Design review of the part built by this model. Coordinates are the model's own, in mm. Face numbers are marked on the shaded views. A direction names the side the tool comes from. Give positions to 0.01 mm unless a question says otherwise; leave off trailing zeros. Order: outer loops, then holes, each group sorted by start corner. A loop starts at its lowest first (then second) coordinate and runs counter-clockwise, first axis right, second up. Notation, with made-up numbers: (29, 4.25) -> (47, 4.25) arc R25 cw to (47, 32.25) -> close; hole circle Ø4 at (62, 17.5). An arc over 180 degrees is marked (long way). One line per item, written item: value. Start each with the question number.
1) The part is to be moulded in two halves that separate along X. For the marked faces 1, 2, 3 and 4, say which applies: released by +X, released by -X, zero draft, split by the parting line, or undercut.
2) Consider section A-A (x = -0.25). State the section outline as (y, z) points.
3) Consider section C-C (z = 3.5). State the section outline as (x, y) points (3 decimals), plus the area to 3 significant figures.
4) Consider section D-D (z = 23.5). State the section outline as (x, y) points (3 decimals).
5) Wall thickness on line 1 along X through (y, z) = (9, 1.75); line 2 along Z through (x, y) = (8.25, 25); line 3 along Y through (x, z) = (0.5, 7.25): over which ranges is each line inside the solid? List them lowest first. Write a range as from..to.
6) Tool access review of the marked faces 5 and 6: name each direction out of +Z, -Z, +X, -X, +Y, -Y from which nothing blocks a thin tool from reaching the whole face with its end or side.
7) For pin 1 (10 mm diameter, centred on x = 1.5, y = 11, fed in from +Z); pin 2 (1.1 mm diameter, centred on x = 11, z = 27, fed in from -Y) (3 decimals); pin 3 (1.9 mm diameter, centred on x = -4.5, z = 28, fed in from +Y) (3 decimals), all flat-tipped, find the tip position at first contact; note any pin that passes through.
8) Consider section B-B (y = 2.95). State the section outline as (x, z) points, plus the area to 3 significant figures.
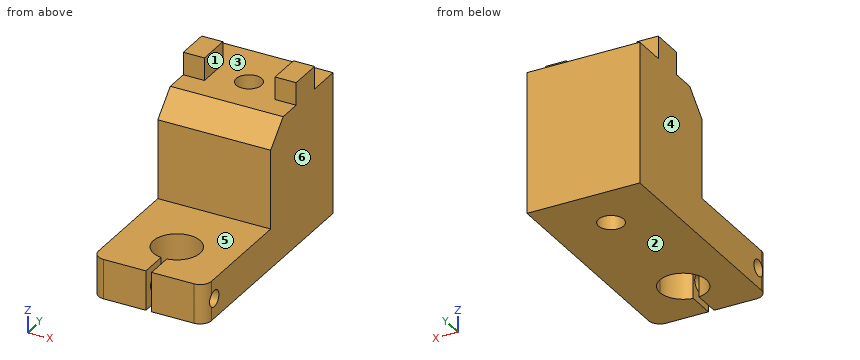
from build123d import *

# Parameters (mm, degrees)
F1_DEPTH    = 7
F2_R        = 1.45
F3_DEPTH    = 25
F4_T1_DEPTH = 17
F5_DEPTH    = 25
F0_W        = 3.75
F0_H        = 5.9
F6_DEPTH    = 29
F7_SIZE     = 4


# Not quite as in the source:
# - a fillet or chamfer that OpenCascade refuses, or shapes differently, is made with other operations: its cross-section is extruded or revolved along the edge and cut away or added
# - a feature names something its author has since deleted; it is built from what else it names


with BuildPart() as f1:
    # F0 (on Top) → F1 (new body)
    with BuildSketch(Plane.XY):
        Polygon((-6.5963959517, 29.175), (-6.5963959517, 21), (13.4036040483, 21), (13.4036040483, 29.175), (9.6536040483, 29.175), (9.6536040483, 35.075), (13.4036040483, 35.075), (13.4036040483, 41), (-6.5963959517, 41), (-6.5963959517, 35.075), (-2.8463959517, 35.075), (-2.8463959517, 29.175), align=None)
        with BuildLine():
            ThreePointArc((1.1536040483, 32.125), (3.4036040483, 34.375), (5.6536040483, 32.125))
            ThreePointArc((5.6536040483, 32.125), (3.4036040483, 29.875), (1.1536040483, 32.125))
        make_face(mode=Mode.SUBTRACT)
        with BuildLine():
            Line((-6.5963959517, 21), (-6.5963959517, 0))
            Line((-6.5963959517, 0), (2.9036040483, 0))
            Line((2.9036040483, 0), (2.9036040483, 4.880230589))
            ThreePointArc((2.9036040483, 4.880230589), (0.6515593539, 12.1062437123), (7.5536040483, 9))
            ThreePointArc((7.5536040483, 9), (6.5098477606, 6.2479553056), (3.9036040483, 4.880230589))
            Line((3.9036040483, 4.880230589), (3.9036040483, 0))
            Line((3.9036040483, 0), (13.4036040483, 0))
            Line((13.4036040483, 0), (13.4036040483, 21))
            Line((13.4036040483, 21), (-6.5963959517, 21))
        make_face()
    extrude(amount=F1_DEPTH)

    # F2 (on face) → F3 (cut)
    with BuildSketch(Plane.YZ.offset(13.4036040483)):
        with Locations((2.95, 3.5)):
            Circle(F2_R)
    extrude(amount=-F3_DEPTH, mode=Mode.SUBTRACT)

    # F4: fillet of radius 2 on 2 edges, made by hand

    # F4_s2 → F4_t1 (cut)
    with BuildSketch(Plane.XY.offset(-5)):
        with BuildLine():
            ThreePointArc((11.4036040483, 0), (12.8178176107, 0.5857864376), (13.4036040483, 2))
            Line((13.4036040483, 2), (13.4036040483, 0))
            Line((13.4036040483, 0), (11.4036040483, 0))
        make_face()
        with BuildLine():
            ThreePointArc((-6.5963959517, 2), (-6.010609514, 0.5857864376), (-4.5963959517, 0))
            Line((-4.5963959517, 0), (-6.5963959517, 0))
            Line((-6.5963959517, 0), (-6.5963959517, 2))
        make_face()
    extrude(amount=F4_T1_DEPTH, mode=Mode.SUBTRACT)

    # F0 (on Top) → F5 (join)
    with BuildSketch(Plane.XY):
        Polygon((-6.5963959517, 29.175), (-6.5963959517, 21), (13.4036040483, 21), (13.4036040483, 29.175), (9.6536040483, 29.175), (9.6536040483, 35.075), (13.4036040483, 35.075), (13.4036040483, 41), (-6.5963959517, 41), (-6.5963959517, 35.075), (-2.8463959517, 35.075), (-2.8463959517, 29.175), align=None)
        with BuildLine():
            ThreePointArc((1.1536040483, 32.125), (3.4036040483, 34.375), (5.6536040483, 32.125))
            ThreePointArc((5.6536040483, 32.125), (3.4036040483, 29.875), (1.1536040483, 32.125))
        make_face(mode=Mode.SUBTRACT)
    extrude(amount=F5_DEPTH)

    # F0 (on Top) → F6 (join)
    with BuildSketch(Plane.XY):
        with Locations((-4.7213959517, 32.125)):
            Rectangle(F0_W, F0_H)
        with Locations((11.5286040483, 32.125)):
            Rectangle(F0_W, F0_H)
    extrude(amount=F6_DEPTH)

    # F7
    f7_edges = [f1.edges().sort_by_distance(p)[0] for p in [
        (3.403604, 21, 25),
    ]]
    chamfer(f7_edges, length=F7_SIZE)


solid = f1.part
Checked values:
1. face 1: undercut
1. face 2: zero draft
1. face 3: undercut
1. face 4: released by -X
2. outline: (0, 0) -> (7.03, 0) -> (7.03, 7) -> (0, 7) -> close; (10.97, 0) -> (41, 0) -> (41, 25) -> (25, 25) -> (21, 21) -> (21, 7) -> (10.97, 7) -> close; hole circle Ø2.9 at (2.95, 3.5)
3. outline: (-6.596, 4.4) -> (2.904, 4.4) -> (2.904, 4.88) arc R4.15 cw (long way) to (3.904, 4.88) -> (3.904, 4.4) -> (13.404, 4.4) -> (13.404, 41) -> (-6.596, 41) -> close; (-6.533, 1.5) arc R2 ccw to (-4.596, 0) -> (2.904, 0) -> (2.904, 1.5) -> close; (3.904, 0) -> (11.404, 0) arc R2 ccw to (13.34, 1.5) -> (3.904, 1.5) -> close; hole circle Ø4.5 at (3.404, 32.125)
3. area: 688 mm^2
4. outline: (-6.596, 23.5) -> (13.404, 23.5) -> (13.404, 41) -> (-6.596, 41) -> close; hole circle Ø4.5 at (3.404, 32.125)
5. line 1: x = -6.6..-0.75, 7.55..13.4
5. line 2: z = 0..25
5. line 3: y = 21..41
6. face 5: +Z, +X, -X, -Y
6. face 6: +Z, -Z, +X, +Y, -Y
7. pin 1: stops at z = 7
7. pin 2: stops at y = 29.175
7. pin 3: stops at y = 35.075
8. outline: (-6.6, 0) -> (2.9, 0) -> (2.9, 2.05) -> (-6.6, 2.05) -> close; (-6.6, 4.95) -> (2.9, 4.95) -> (2.9, 7) -> (-6.6, 7) -> close; (3.9, 0) -> (13.4, 0) -> (13.4, 2.05) -> (3.9, 2.05) -> close; (3.9, 4.95) -> (13.4, 4.95) -> (13.4, 7) -> (3.9, 7) -> close
8. area: 77.9 mm^2
